Source: CAD feature listing. Evaluate the final solid. Frame: model axes, mm. Face numbers are marked on the shaded views. A direction names the side the tool comes from. Round coordinates to 2 decimals unless told otherwise and drop trailing zeros. Loops run counter-clockwise (first coordinate to the right, second up) from the corner with the lowest first, then second, coordinate; pieces in that order, holes last. Notation, with made-up numbers: (59, 27.25) -> (102, 27.25) arc R27 cw to (102, 58.25) -> close; hole circle Ø10 at (-32, 23.25). An arc over 180 degrees is marked (long way). Put each result on its own line as item: value. Start each with the question number.
1. Material intervals for L1, parallel to Z at x = 71.5, y = -2; L2, parallel to X at y = 37.5, z = -51; L3, parallel to X at y = 35.5, z = -15.5, sorted ascending.
2. Cut plane D-D (z = -43). Return the cut outline in (x, y).
3. Cut plane B-B (z = 10). Return the cut outline in (x, y), then the cut area to 3 significant figures.
4. Draft query along Y for the marked faces 1, 2 and 3. Return one class per face: pulls with the +Y half, pulls with the -Y half, needs draft (parallel to the pull), parting line crosses it, or undercut.
5. Set-up query: the marked faces 4, 5 and 6. Return all of +Z, -Z, +X, -X, +Y, -Y with unobstructed straight access to the full face (end or side cutting, diameter ignored); none if empty.
6. Contact query for flat-ended pins moving along their axis: pin 1 (8 mm diameter, centred on x = 37.5, y = 25.5, fed in from +Z); pin 2 (1.5 mm diameter, centred on y = 16.5, z = -37.5, fed in from +X); pin 3 (8 mm diameter, centred on x = 89.5, y = -39.5, fed in from +Z). Output: stop coordinate, or through.
7. Cut plane C-C (y = 43). Return the cut outline in (x, z), then the cut area to 3 significant figures.
8. Cut plane A-A (x = 96). Return the cut outline in (y, z).
```python
from build123d import *

# Parameters (mm, degrees)
REVOLVE1_ANGLE = 270


with BuildPart() as part:
    # Sketch1 → Revolve1 (revolve)
    with BuildSketch(Plane.XY):
        Polygon((120, 0), (0, 0), (0, 25), (40, 25), (40, 40), (80, 40), (80, 55), (120, 55), (120, 70), (160, 70), (160, 65), (125, 65), (125, 50), (85, 50), (85, 35), (45, 35), (45, 20), (120, 20), align=None)
    revolve(axis=Axis((120, 0, 0), (-1, 0, 0)), revolution_arc=REVOLVE1_ANGLE)


solid = part.part
```
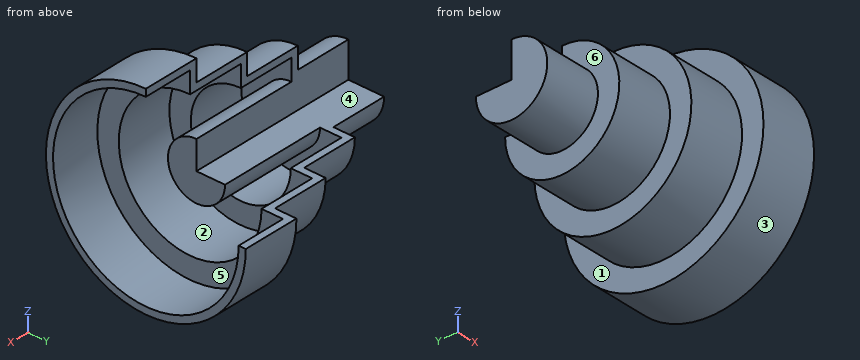
Solution:
1. L1: z = -39.95 to -34.94, -19.9 to 19.9, 34.94 to 39.95
1. L2: x = 120 to 125
1. L3: x = 40 to 85
2. outline: (80, -34.29) -> (120, -34.29) -> (120, -55.24) -> (160, -55.24) -> (160, -48.74) -> (125, -48.74) -> (125, -25.51) -> (85, -25.51) -> (85, 25.51) -> (125, 25.51) -> (125, 48.74) -> (160, 48.74) -> (160, 55.24) -> (120, 55.24) -> (120, 34.29) -> (80, 34.29) -> close
3. outline: (0, -22.91) -> (40, -22.91) -> (40, -38.73) -> (80, -38.73) -> (80, -54.08) -> (120, -54.08) -> (120, -69.28) -> (160, -69.28) -> (160, -64.23) -> (125, -64.23) -> (125, -48.99) -> (85, -48.99) -> (85, -33.54) -> (45, -33.54) -> (45, -17.32) -> (120, -17.32) -> (120, 0) -> (0, 0) -> close
3. area: 3,150 mm^2
4. face 1: needs draft
4. face 2: undercut
4. face 3: parting line crosses it
5. face 4: +Z, +X, -X, +Y
5. face 5: +X
5. face 6: -X
6. pin 1: stops at z = 0
6. pin 2: stops at x = 85
6. pin 3: stops at z = 42.01
7. outline: (80, -34.29) -> (120, -34.29) -> (120, -55.24) -> (160, -55.24) -> (160, -48.74) -> (125, -48.74) -> (125, -25.51) -> (85, -25.51) -> (85, 0) -> (80, 0) -> close
7. area: 855 mm^2
8. outline: (0, 0) -> (0, 20) arc R20 ccw (long way) to (20, 0) -> close; (0, 50) -> (0, 55) arc R55 ccw (long way) to (55, 0) -> (50, 0) arc R50 cw (long way) to start
